Design review of the part built by this model. Coordinates are the model's own, in mm. Coordinates: 2 decimals unless noted, no trailing zeros. Write each loop counter-clockwise with the first axis right and the second up, starting at its lowest first coordinate (ties: lowest second). Pieces come first, ordered by that corner, then holes.
Q1. Add section C-C, the plane z = -4.75. Give the boundary of the cut face in (x, y).
Q2. Clearance check with flat-ended pins moving along their axes: pin 1 Ø3 at (y, z) = (0.5, -3) entering from +X; pin 2 Ø1 at (x, z) = (-1, -4) entering from +Y; pin 3 Ø2.5 at (y, z) = (0, 0) entering from -X. State where each tip first meets the part, or that it passes through.
Q3. Add section D-D, the plane z = 1. Give the boundary of the cut face in (x, y), plus the area to 3 significant figures.
Q4. Add section A-A, the plane y = -0.5. Give the boundary of the cut face in (x, z), plus the area to 3 significant figures.
Q5. The part is to be moulded in two halves that separate along X. For faces 1 (the face through (0, -2, -5)), 2 (the face through (-1.5, 0.07, -4.96)), say which applies: +X half, -X half, draft (parallel to the pull), parting line (faces both ways), or undercut.
Q6. To check wall thickness, follow probe 1 along Y at (x, z) = (0, -5.1); probe 2 along X at (y, z) = (-1.1, -6). State the ranges of each line that lie inside material, in increasing order.
Q7. Add section B-B, the plane x = 1.3. Give the boundary of the cut face in (y, z), plus the area to 3 significant figures.
Autodesk Inventor part; units mm, degrees
ref_plane "YZ Plane" through (0, 0, 0) normal (1, 0, 0) x (0, 1, 0)
ref_plane "XZ Plane" through (0, 0, 0) normal (0, 1, 0) x (-1, 0, 0)
ref_plane "XY Plane" through (0, 0, 0) normal (0, 0, 1) x (1, 0, 0)
sketch "Sketch1" plane through (0, 0, 0) normal (0, 1, 0) x (-1, 0, 0)
  circle A0 centre (0, 0) radius 2.5
  line L0 (0, -3.5) -> (0, 3.5)
  line L1 (0, 2.5) -> (0, -2.5)
  dimension "d0" = 5
revolve "Revolution1" add sketch "Sketch1" angle 360 about axis through (0, 0, 0) along (0, 0, 1) picked at (0.5196, 0.6515) contours A0 L0
sketch "Sketch2" plane through (0, 0, 0) normal (0, 0, 1) x (1, 0, 0)
  circle A0 centre (0, 0) radius 2
  circle A1 centre (0, 0) radius 1.5
  dimension "d2" = 4
  dimension "d3" = 3
extrude "Extrusion1" add sketch "Sketch2" against normal blind 8
sketch "Sketch3" plane through (0, 0, 0) normal (1, 0, 0) x (0, 1, 0)
  circle A0 centre (0, 0) radius 1.5
  dimension "d6" = 3
extrude "Extrusion2" cut sketch "Sketch3" against normal through all
fillet "Fillet1" radius 1.5 1 edges at (0, -1.5, 0)
properties part number "P_snap_001" material "PC/ABS Plastic"
Here are the results:
1. outline: circle Ø4 at (0, 0); hole circle Ø3 at (0, 0)
2. pin 1: stops at x = 2
2. pin 2: stops at y = 1.94
2. pin 3: stops at x = -0.67
3. outline: (-2, -1.12) arc R2.29 ccw (long way) to (-2, 1.12) - (-1.5, 1.12) arc R1.12 cw to (-1.5, -1.12) - close
3. area: 13.0 mm2
4. outline: (-2, -1.41) arc R2.45 ccw to (-1.94, -1.5) - (-1.94, -8) - (-1.41, -8) - (-1.41, -2) arc R2.45 ccw to (1.41, -2) - (1.41, -8) - (1.94, -8) - (1.94, -1.5) arc R2.45 ccw (long way) to (-2, 1.41) - (-1.5, 1.41) arc R1.41 cw to (-1.5, -1.41) - close
4. area: 19.9 mm2
5. face 1: parting line
5. face 2: undercut
6. probe 1: y = -2 to -1.5, 1.5 to 2
6. probe 2: x = -1.67 to -1.02, 1.02 to 1.67
7. outline: (-1.52, -8) - (-0.75, -8) - (-0.75, -2) arc R2.14 ccw to (0.75, -2) - (0.75, -8) - (1.52, -8) - (1.52, -1.5) arc R2.14 ccw (long way) to (-1.52, -1.5) - close
7. area: 23.9 mm2
